Geometry: final body of the model. Coordinates: model frame, mm. A direction names the side the tool comes from. Coordinates: 2 decimals unless noted, no trailing zeros. Write each loop counter-clockwise with the first axis right and the second up, starting at its lowest first coordinate (ties: lowest second). Pieces come first, ordered by that corner, then holes.
from build123d import *

# Parameters (mm, degrees)
MAIN_FEATURES_SKETCH_R           = 24.5
MAIN_FEATURES_SKETCH_R_2         = 15.75
MAIN_FEATURES_SKETCH_R_3         = 12.7
MAIN_FEATURES_SKETCH_R_4         = 13.9
OUTER_RING_DEPTH                 = 4
MAIN_FEATURES_SKETCH_3_R         = 15.75
MAIN_FEATURES_SKETCH_3_R_2       = 13.9
MAIN_FEATURES_SKETCH_3_R_3       = 12.7
INNER_RING_DEPTH                 = 3
MAIN_FEATURES_SKETCH_4_R         = 13.9
MAIN_FEATURES_SKETCH_4_R_2       = 12.7
SUPPORT_RING_DEPTH               = 6
MAIN_FEATURES_SKETCH_5_R         = 3.2639
MAIN_FEATURES_SKETCH_5_W         = 101.6
MAIN_FEATURES_SKETCH_5_H         = 4
MAIN_FEATURES_SKETCH_5_W_2       = 69.85
MAIN_FEATURES_SKETCH_5_W_3       = 19.05
MAIN_FEATURES_SKETCH_5_W_4       = 12.7
PLATE_DEPTH                      = 4
MAIN_FEATURES_SKETCH_6_W         = 12.7
MAIN_FEATURES_SKETCH_6_H         = 4
MAIN_FEATURES_SKETCH_6_W_2       = 69.85
LEDGE_DEPTH                      = 10
F_1_4_20_TAPPED_HOLE1_AT_2_COUNT = 2
F_1_4_20_TAPPED_HOLE1_AT_2_PITCH = 25.4
F_1_4_20_TAPPED_HOLE1_AT_3_COUNT = 2
F_1_4_20_TAPPED_HOLE1_AT_3_PITCH = 76.2
F_1_4_20_TAPPED_HOLE1_AT_4_COUNT = 2
F_1_4_20_TAPPED_HOLE1_AT_4_PITCH = 50.8
FILLET1_R                        = 1
CHAMFER1_SIZE                    = 0.2


with BuildPart() as part:
    # main_features_sketch → outer_ring (new body)
    with BuildSketch(Plane.XY):
        with Locations((-10, 0)):
            Circle(MAIN_FEATURES_SKETCH_R)
        with Locations((-10, 0)):
            Circle(MAIN_FEATURES_SKETCH_R_2, mode=Mode.SUBTRACT)
        with Locations((-10, 0)):
            Circle(MAIN_FEATURES_SKETCH_R_2)
        with Locations((-10, 0)):
            Circle(MAIN_FEATURES_SKETCH_R_3, mode=Mode.SUBTRACT)
        with Locations((-10, 0)):
            Circle(MAIN_FEATURES_SKETCH_R_4)
        with Locations((-10, 0)):
            Circle(MAIN_FEATURES_SKETCH_R_3, mode=Mode.SUBTRACT)
    extrude(amount=OUTER_RING_DEPTH)

    # main_features_sketch<3> → inner_ring (add)
    with BuildSketch(Plane.XY):
        with Locations((-10, 0)):
            Circle(MAIN_FEATURES_SKETCH_3_R)
        with Locations((-10, 0)):
            Circle(MAIN_FEATURES_SKETCH_3_R_2, mode=Mode.SUBTRACT)
        with Locations((-10, 0)):
            Circle(MAIN_FEATURES_SKETCH_3_R_2)
        with Locations((-10, 0)):
            Circle(MAIN_FEATURES_SKETCH_3_R_3, mode=Mode.SUBTRACT)
    extrude(amount=-INNER_RING_DEPTH)

    # main_features_sketch<4> → support_ring (add)
    with BuildSketch(Plane.XY):
        with Locations((-10, 0)):
            Circle(MAIN_FEATURES_SKETCH_4_R)
        with Locations((-10, 0)):
            Circle(MAIN_FEATURES_SKETCH_4_R_2, mode=Mode.SUBTRACT)
    extrude(amount=SUPPORT_RING_DEPTH)

    # groove_sketch → groove (revolve, cut)
    with BuildSketch(Plane(origin=(-10, 0, 0), x_dir=(0, 0, -1), z_dir=(1, 0, 0)), mode=Mode.PRIVATE) as groove_sk:
        Polygon((2.35, 15.75), (1.65, 15.05), (0.95, 15.75), align=None)
    revolve(groove_sk.sketch.rotate(Axis((-10, 0, 4), (0, 0, -1)), 90), axis=Axis((-10, 0, 4), (0, 0, -1)), mode=Mode.SUBTRACT)

    # main_features_sketch<5> → plate (add)
    with BuildSketch(Plane.XY):
        with BuildLine():
            add(Edge.make_bspline(
                [(-32.6, -60.8), (-32.6, -39.723627729), (-28.738697218, -22.987442245), (-33.489342322, -6.96425138)],
                knots=[0, 0, 0, 0, 1, 1, 1, 1], degree=3))
            Line((-32.6, -60.8), (37.25, -60.8))
            Line((37.25, -60.8), (56.3, -60.8))
            Line((56.3, -60.8), (69, -60.8))
            Line((69, -60.8), (69, -35.4))
            add(Edge.make_bspline(
                [(69, -35.4), (69, -15.705164825), (20.577875926, -1.371414224), (10.248802697, 13.792606329)],
                knots=[0, 0, 0, 0, 1, 1, 1, 1], degree=3))
            ThreePointArc((10.248802697, 13.792606329), (13.413091061, 7.216451134), (14.5, 0))
            ThreePointArc((14.5, 0), (-6.481398494, -24.246019126), (-33.489342322, -6.96425138))
        make_face()
        with Locations((-19.9, -48.1)):
            Circle(MAIN_FEATURES_SKETCH_5_R, mode=Mode.SUBTRACT)
        with Locations((5.5, -48.1)):
            Circle(MAIN_FEATURES_SKETCH_5_R, mode=Mode.SUBTRACT)
        with Locations((30.9, -48.1)):
            Circle(MAIN_FEATURES_SKETCH_5_R, mode=Mode.SUBTRACT)
        with Locations((56.3, -48.1)):
            Circle(MAIN_FEATURES_SKETCH_5_R, mode=Mode.SUBTRACT)
        with Locations((18.2, -62.8)):
            Rectangle(MAIN_FEATURES_SKETCH_5_W, MAIN_FEATURES_SKETCH_5_H)
        with Locations((2.325, -62.8)):
            Rectangle(MAIN_FEATURES_SKETCH_5_W_2, MAIN_FEATURES_SKETCH_5_H)
        with Locations((46.775, -62.8)):
            Rectangle(MAIN_FEATURES_SKETCH_5_W_3, MAIN_FEATURES_SKETCH_5_H)
        with Locations((62.65, -62.8)):
            Rectangle(MAIN_FEATURES_SKETCH_5_W_4, MAIN_FEATURES_SKETCH_5_H)
    extrude(amount=PLATE_DEPTH)

    # main_features_sketch<6> → ledge (add)
    with BuildSketch(Plane.XY):
        with Locations((62.65, -62.8)):
            Rectangle(MAIN_FEATURES_SKETCH_6_W, MAIN_FEATURES_SKETCH_6_H)
        with Locations((2.325, -62.8)):
            Rectangle(MAIN_FEATURES_SKETCH_6_W_2, MAIN_FEATURES_SKETCH_6_H)
    extrude(amount=-LEDGE_DEPTH)

    # Sketch2 → 1/4-20 Tapped Hole1 (revolve, cut)
    with BuildSketch(Plane(origin=(56.3, -29.05, 4), x_dir=(0, -1, 0), z_dir=(1, 0, 0))):
        Polygon((0, 0), (0, 4), (3.302, 4), (2.5527, 3.2507), (2.5527, 0.7493), (3.302, 0), align=None)
    f_1_4_20_tapped_hole1 = revolve(axis=Axis((56.3, -29.05, 10.35), (0, 0, -1)), mode=Mode.SUBTRACT)

    # 1/4-20 Tapped Hole1 at 2: 1/4-20 Tapped Hole1 ×2
    with Locations(*[(-i * F_1_4_20_TAPPED_HOLE1_AT_2_PITCH, 0, 0) for i in range(1, F_1_4_20_TAPPED_HOLE1_AT_2_COUNT)]):
        add(f_1_4_20_tapped_hole1, mode=Mode.SUBTRACT)

    # 1/4-20 Tapped Hole1 at 3: 1/4-20 Tapped Hole1 ×2
    with Locations(*[(-i * F_1_4_20_TAPPED_HOLE1_AT_3_PITCH, 0, 0) for i in range(1, F_1_4_20_TAPPED_HOLE1_AT_3_COUNT)]):
        add(f_1_4_20_tapped_hole1, mode=Mode.SUBTRACT)

    # 1/4-20 Tapped Hole1 at 4: 1/4-20 Tapped Hole1 ×2
    with Locations(*[(-i * F_1_4_20_TAPPED_HOLE1_AT_4_PITCH, 0, 0) for i in range(1, F_1_4_20_TAPPED_HOLE1_AT_4_COUNT)]):
        add(f_1_4_20_tapped_hole1, mode=Mode.SUBTRACT)

    # Fillet1
    fillet1_edges = [part.edges().sort_by_distance(p)[0] for p in [
        (69, -64.8, -3),
        (-32.6, -64.8, -3),
        (56.3, -64.8, -5),
        (56.3, -60.8, -5),
        (69, -60.8, -5),
        (37.25, -64.8, -5),
        (-32.6, -60.8, -5),
        (37.25, -60.8, -5),
    ]]
    fillet(fillet1_edges, radius=FILLET1_R)

    # Chamfer1
    chamfer1_edges = [part.edges().sort_by_distance(p)[0] for p in [
        (-23.9, 0, 6),
        (-22.7, 0, 6),
        (-25.75, 0, -3),
        (-22.7, 0, -3),
        (-23.1639, -48.1, 0),
        (-23.1639, -48.1, 4),
        (2.2361, -48.1, 0),
        (2.2361, -48.1, 4),
        (27.6361, -48.1, 0),
        (27.6361, -48.1, 4),
        (53.0361, -48.1, 0),
        (53.0361, -48.1, 4),
        (68.707106781, -61.092893219, -10),
        (62.65, -60.8, -10),
        (56.592893219, -61.092893219, -10),
        (56.3, -62.8, -10),
        (56.592893219, -64.507106781, -10),
        (62.65, -64.8, -10),
        (68.707106781, -64.507106781, -10),
        (69, -62.8, -10),
        (-32.307106781, -61.092893219, -10),
        (-32.6, -62.8, -10),
        (-32.307106781, -64.507106781, -10),
        (2.325, -64.8, -10),
        (36.957106781, -64.507106781, -10),
        (37.25, -62.8, -10),
        (36.957106781, -61.092893219, -10),
        (2.325, -60.8, -10),
        (68.707106781, -64.507106781, 4),
        (18.2, -64.8, 4),
        (69, -49.6, 4),
        (-32.307106781, -64.507106781, 4),
        (42.397221588, -8.455112608, 4),
        (42.397221588, -8.455112608, 0),
        (-32.6, -62.3, 4),
        (-20.504144885, 22.133977054, 4),
        (-20.504144885, 22.133977054, 0),
        (-31.34637018, -33.788834835, 4),
        (-31.34637018, -33.788834835, 0),
        (46.775, -64.8, 0),
        (69, -48.6, 0),
        (-32.6, -61.3, 0),
    ]]
    chamfer(chamfer1_edges, length=CHAMFER1_SIZE)


solid = part.part
Item 1: Section B-B, the plane y = -48.1. State how many separate pieces and enclosed holes the cut face has, plus the area to 3 significant figures.
Derived:
separate pieces: 5
enclosed holes: 0
area: 300 mm2
Item 2: Pull-direction query (X, two-part tool) for faces 5 (the cylindrical face through (57.8, -51, 2)), 6 (the cylindrical face through (2.84, -5.32, 4.89)), 7 (the flat face through (18, -29, 4)), 8 (the cylindrical face through (-20.1, -7.7, 1.4)); classes: released by +X, released by -X, zero draft, split by the parting line, or undercut.
Derived:
face 5: undercut
face 6: split by the parting line
face 7: zero draft
face 8: undercut
Item 3: Set-up query: faces 1 (the flat face through (-32.6, -63, -3)), 2 (the flat face through (-16, 12, -3)), 3 (the cylindrical face through (58.565, -30.228, 2.018)), 4 (the cylindrical face through (5.023, 4.731, -0.468)). Return all of +Z, -Z, +X, -X, +Y, -Y with unobstructed straight access to the full face (end or side cutting, diameter ignored); none if empty.
Derived:
face 1: +Z, -Z, -X, -Y
face 2: -Z, +X, -X, +Y
face 3: +Z, -Z
face 4: -Z
Item 4: Material intervals for probe 1 along Y at (x, z) = (5.5, 1.55); probe 2 along Y at (x, z) = (56.3, 1.9); probe 3 along Y at (x, z) = (-19.9, 2.2), sorted ascending.
Derived:
probe 1: y = -64.8 to -51.36, -44.84 to -31.6, -26.5 to 18.97
probe 2: y = -64.8 to -51.36, -44.84 to -31.6, -26.5 to -17.44
probe 3: y = -64.8 to -51.36, -44.84 to -31.6, -26.5 to -7.95, 7.95 to 22.41
Item 5: Section A-A, the plane z = -7.75. Output: boundary loops of the cut face in (x, y).
Derived:
outline: (-32.6, -63.8) arc R1 ccw to (-31.6, -64.8) - (36.25, -64.8) arc R1 ccw to (37.25, -63.8) - (37.25, -61.8) arc R1 ccw to (36.25, -60.8) - (-31.6, -60.8) arc R1 ccw to (-32.6, -61.8) - close; (56.3, -63.8) arc R1 ccw to (57.3, -64.8) - (68, -64.8) arc R1 ccw to (69, -63.8) - (69, -61.8) arc R1 ccw to (68, -60.8) - (57.3, -60.8) arc R1 ccw to (56.3, -61.8) - close
Item 6: Pin query (flat end, axial travel): pin 1 (8 mm diameter, centred on y = 13.5, z = -5, fed in from -X); pin 2 (6 mm diameter, centred on x = 5.5, y = -29.05, fed in from -Z); pin 3 (1.5 mm diameter, centred on y = -62, z = -5, fed in from -X); pin 4 (4 mm diameter, centred on x = 30.9, y = -48.1, fed in from -Z). Return the tip coordinate at first contact, or that it passes through.
Derived:
pin 1: stops at x = -22.04
pin 2: stops at z = 0.3
pin 3: stops at x = -32.6
pin 4: passes through
